```python
from build123d import *

# Parameters (mm, degrees)
CROQUIS1_W              = 6.35
CROQUIS1_H              = 40
SALIENTE_EXTRUIR1_DEPTH = 130
CROQUIS2_W              = 6.35
CROQUIS2_H              = 40
SALIENTE_EXTRUIR2_DEPTH = 30
CHAFL_N1_SIZE           = 1


with BuildPart() as part:
    # Croquis1 → Saliente-Extruir1 (new body)
    with BuildSketch(Plane.XY):
        Rectangle(CROQUIS1_W, CROQUIS1_H)
    extrude(amount=SALIENTE_EXTRUIR1_DEPTH)

    # Croquis2 → Saliente-Extruir2 (add)
    with BuildSketch(Plane(origin=(3.175, 0, 0), x_dir=(0, 0, -1), z_dir=(1, 0, 0))):
        with Locations((-33.175, 0)):
            Rectangle(CROQUIS2_W, CROQUIS2_H)
    extrude(amount=SALIENTE_EXTRUIR2_DEPTH)

    # Chaflán1
    chafl_n1_edges = [part.edges().sort_by_distance(p)[0] for p in [
        (3.175, 0, 130),
        (3.175, 20, 15),
        (3.175, -20, 15),
        (18.175, 20, 30),
        (3.175, 0, 36.35),
        (18.175, 20, 36.35),
        (18.175, -20, 36.35),
        (3.175, 0, 30),
        (18.175, -20, 30),
        (33.175, 20, 33.175),
        (33.175, 0, 36.35),
        (33.175, -20, 33.175),
        (33.175, 0, 30),
        (-3.175, 0, 130),
        (3.175, 0, 0),
        (-3.175, 0, 0),
        (-3.175, 20, 65),
        (3.175, 20, 83.175),
        (3.175, -20, 83.175),
        (-3.175, -20, 65),
    ]]
    chamfer(chafl_n1_edges, length=CHAFL_N1_SIZE)


solid = part.part
```
Model file for the job. Use its own axes, mm. A direction names the side the tool comes from. Give positions to 0.01 mm unless a question says otherwise; leave off trailing zeros. Loops run counter-clockwise (first coordinate to the right, second up) from the corner with the lowest first, then second, coordinate; pieces in that order, holes last. Notation, with made-up numbers: (-29, 85.25) -> (4, 85.25) arc R18 ccw to (4, 98.25) -> close; hole circle Ø3 at (31, -11). An arc over 180 degrees is marked (long way). Write each question's results on one line, items separated by ' | '.
(1) Cut at C-C on x = 14.5. List the corners of the cut face in (y, z), and give its area (3 significant figures).
Geometry results:
outline: (-20, 31) -> (-19, 30) -> (19, 30) -> (20, 31) -> (20, 35.35) -> (19, 36.35) -> (-19, 36.35) -> (-20, 35.35) -> close | area: 252 mm²
(2) Probe line 1 along X through (y, z) = (13.5, 49) (3 decimals); line 2 along Z through (x, y) = (22, 12); line 3 along Z through (x, y) = (3, 7) (3 decimals). List the from-to ranges inside material, lowest first.
Geometry results:
line 1: x = -3.175 to 3.175 | line 2: z = 30 to 36.35 | line 3: z = 0.825 to 129.175
(3) Tool access for faces 1 (the flat face through (0, -20, 65)), 2 (the flat face through (3.175, 0, 15)), 3 (the flat face through (3.175, 0, 83)): list every direction of +Z, -Z, +X, -X, +Y, -Y with a clear straight run to the whole face (end or side of a thin tool).
Geometry results:
face 1: +Z, -Z, +X, -X, -Y | face 2: -Z, +X, +Y, -Y | face 3: +Z, +X, +Y, -Y
(4) Cut at B-B on y = -14.5. List the corners of the cut face in (x, z) (3 decimals).
Geometry results:
outline: (-3.175, 1) -> (-2.175, 0) -> (2.175, 0) -> (3.175, 1) -> (3.175, 29) -> (4.175, 30) -> (32.175, 30) -> (33.175, 31) -> (33.175, 35.35) -> (32.175, 36.35) -> (4.175, 36.35) -> (3.175, 37.35) -> (3.175, 129) -> (2.175, 130) -> (-2.175, 130) -> (-3.175, 129) -> close
(5) Flat gauge pins, fed straight in: pin 1 Ø3 at (y, z) = (10, 82) entering from +X (3 decimals); pin 2 Ø8 at (x, z) = (10, 41.5) entering from -Y; pin 3 Ø14 at (x, y) = (16, -5) entering from -Z; pin 4 Ø8.5 at (x, y) = (12, -7) entering from +Z. Where does each tip first touch, or does it go through?
Geometry results:
pin 1: stops at x = 3.175 | pin 2: passes through | pin 3: stops at z = 30 | pin 4: stops at z = 36.35
(6) Cut at A-A on z = 45. List the corners of the cut face in (x, y) (3 decimals).
Geometry results:
outline: (-3.175, -19) -> (-2.175, -20) -> (2.175, -20) -> (3.175, -19) -> (3.175, 19) -> (2.175, 20) -> (-2.175, 20) -> (-3.175, 19) -> close
